The listing builds one solid part. Answer for the finished solid, in the listing's coordinates (mm). A direction names the side the tool comes from. Coordinates: 2 decimals unless noted, no trailing zeros. Order: outer loops, then holes, each group sorted by start corner. A loop starts at its lowest first (then second) coordinate and runs counter-clockwise, first axis right, second up. Notation, with made-up numbers: (-15.5, -28) -> (43.5, -28) arc R32 ccw to (43.5, 7) -> close; hole circle Ø5 at (11, 12). An arc over 180 degrees is marked (long way). Write each question's results on one line, items separated by ' | '. Start each with the question number.
(1) A tool of negligible diameter and unlimited length cuts with its end or side. For faces 4 (the face through (16, -21, 10)), 5 (the face through (9.15, -4.86, 15.1)), 6 (the face through (16.9, 4.14, 9.86)), from which of +Z, -Z, +X, -X, +Y, -Y can it reach the whole face along a straight path? Write none if from no direction.
(2) The part is cut by section C-C, the plane z = 10. Count the separate pieces of the cut face and the enclosed holes in it, then the cut area to 3 significant figures.
(3) Straight lines are drawn through the part: L1, parallel to X at y = 1, z = 2; L2, parallel to X at y = -7, z = 14; L3, parallel to Y at x = 3.75, z = -2.5. For each, find the intervals that lie inside material, in ascending order.
(4) The part is cut by section B-B, the plane x = 11.5. Give the vertices of the cut face in (y, z), then the cut area to 3 significant figures.
(5) Determine the mould class of faces 1 (the face through (2.768, -9.84, 13.646)), 2 (the face through (14.9, -4.86, 2.67)), 3 (the face through (13, -10, 20)) for opening direction Z: +Z half, -Z half, draft (parallel to the pull), parting line (faces both ways), or undercut.
(6) The part is cut by section A-A, the plane x = 20. Give the vertices of the cut face in (y, z), then the cut area to 3 significant figures.
(7) Given pin 1 (3 mm diameter, centred on x = 8, y = -19, fed in from -Z); pin 2 (5 mm diameter, centred on y = -14, z = 19, fed in from +X); pin 3 (1 mm diameter, centred on x = 20.5, z = 6.5, fed in from -Y), each flat-ended and moving along its own axis, determine where each tip first touches the part or whether it passes through.
```python
from build123d import *

# Parameters (mm, degrees)
SKETCH1_W           = 20
SKETCH1_H           = 20
BOSS_EXTRUDE1_DEPTH = 4
SKETCH2_R           = 3.65
CUT_EXTRUDE1_DEPTH  = 2.5
SKETCH3_R           = 2.25
CUT_EXTRUDE2_DEPTH  = 29.394541729
SKETCH4_W           = 12
SKETCH4_H           = 4
BOSS_EXTRUDE2_DEPTH = 10
SKETCH7_W           = 20
SKETCH7_H           = 4
BOSS_EXTRUDE3_DEPTH = 10
SKETCH8_W           = 8
SKETCH8_H           = 20
BOSS_EXTRUDE4_DEPTH = 5
SKETCH9_W           = 8
SKETCH9_H           = 20
BOSS_EXTRUDE5_DEPTH = 5
SKETCH10_R          = 1.6
CUT_EXTRUDE5_DEPTH  = 41.012498047
SKETCH11_W          = 32
SKETCH11_H          = 32
SKETCH11_W_2        = 20
SKETCH11_H_2        = 20
BOSS_EXTRUDE6_DEPTH = 6
FILLET6_R           = 3
SKETCH13_R          = 1.35
CUT_EXTRUDE7_DEPTH  = 6
FILLET7_R           = 3
FILLET13_R          = 2
FILLET14_SIZE       = 13


with BuildPart() as part:
    # Sketch1 → Boss-Extrude1 (new body)
    with BuildSketch(Plane(origin=(0, 0, 0), x_dir=(0, 0, -1), z_dir=(1, 0, 0))):
        with Locations((-10, -10)):
            Rectangle(SKETCH1_W, SKETCH1_H)
    extrude(amount=BOSS_EXTRUDE1_DEPTH)

    # Sketch2 → Cut-Extrude1 (cut)
    with BuildSketch(Plane(origin=(4, 0, 0), x_dir=(0, 0, -1), z_dir=(1, 0, 0))):
        with Locations((-10, -10)):
            Circle(SKETCH2_R)
    extrude(amount=-CUT_EXTRUDE1_DEPTH, mode=Mode.SUBTRACT)

    # Sketch3 → Cut-Extrude2 (cut, through all)
    with BuildSketch(Plane(origin=(1.5, 0, 0), x_dir=(0, 0, -1), z_dir=(1, 0, 0))):
        with Locations((-10, -10)):
            Circle(SKETCH3_R)
    extrude(amount=-CUT_EXTRUDE2_DEPTH, mode=Mode.SUBTRACT)

    # Sketch4 → Boss-Extrude2 (add)
    with BuildSketch(Plane(origin=(4, 0, 0), x_dir=(0, 0, -1), z_dir=(1, 0, 0))):
        Polygon((-20, 0), (-20, -20), (-16, -20), (-16, -16), (-16, -4), (-16, 0), align=None)
        with Locations((-10, -18)):
            Rectangle(SKETCH4_W, SKETCH4_H)
        Polygon((-4, -16), (-4, -20), (0, -20), (0, -4), (-4, -4), align=None)
        Polygon((0, 0), (-16, 0), (-16, -4), (-4, -4), (0, -4), align=None)
    extrude(amount=BOSS_EXTRUDE2_DEPTH)

    # Sketch7 → Boss-Extrude3 (add)
    with BuildSketch(Plane(origin=(14, 0, 0), x_dir=(0, 0, -1), z_dir=(1, 0, 0))):
        with Locations((-10, -18)):
            Rectangle(SKETCH7_W, SKETCH7_H)
        with Locations((-10, -2)):
            Rectangle(SKETCH7_W, SKETCH7_H)
    extrude(amount=BOSS_EXTRUDE3_DEPTH)

    # Sketch8 → Boss-Extrude4 (add)
    with BuildSketch(Plane(origin=(0, -20, 0), x_dir=(-1, 0, 0), z_dir=(0, -1, 0))):
        with Locations((-20, -10)):
            Rectangle(SKETCH8_W, SKETCH8_H)
    extrude(amount=BOSS_EXTRUDE4_DEPTH)

    # Sketch9 → Boss-Extrude5 (add)
    with BuildSketch(Plane(origin=(0, 0, 0), x_dir=(1, 0, 0), z_dir=(0, 1, 0))):
        with Locations((20, -10)):
            Rectangle(SKETCH9_W, SKETCH9_H)
    extrude(amount=BOSS_EXTRUDE5_DEPTH)

    # Sketch10 → Cut-Extrude5 (cut, through all)
    with BuildSketch(Plane(origin=(0, 0, 0), x_dir=(-1, 0, 0), z_dir=(0, 0, -1))):
        with Locations(Location((-20, 1, 0), (0, 0, 90))):
            Circle(SKETCH10_R)
        with Locations(Location((-20, -21, 0), (0, 0, 90))):
            Circle(SKETCH10_R)
    extrude(amount=-CUT_EXTRUDE5_DEPTH, mode=Mode.SUBTRACT)

    # Sketch11 → Boss-Extrude6 (add)
    with BuildSketch(Plane.ZY):
        with Locations((10, -10)):
            Rectangle(SKETCH11_W, SKETCH11_H)
        with Locations((10, -10)):
            Rectangle(SKETCH11_W_2, SKETCH11_H_2, mode=Mode.SUBTRACT)
    extrude(amount=-BOSS_EXTRUDE6_DEPTH)

    # Fillet6
    fillet6_edges = [part.edges().sort_by_distance(p)[0] for p in [
        (24, -16, 10),
        (24, -4, 10),
        (24, -25, 10),
        (16, -25, 10),
        (24, 5, 10),
        (16, 5, 10),
    ]]
    fillet(fillet6_edges, radius=FILLET6_R)

    # Sketch13 → Cut-Extrude7 (cut)
    with BuildSketch(Plane.ZY):
        with Locations((22.5, -10)):
            Circle(SKETCH13_R)
        with Locations((10, 2.5)):
            Circle(SKETCH13_R)
        with Locations((-2.5, -10)):
            Circle(SKETCH13_R)
        with Locations((10, -22.5)):
            Circle(SKETCH13_R)
    extrude(amount=-CUT_EXTRUDE7_DEPTH, mode=Mode.SUBTRACT)

    # Fillet7
    fillet7_edges = [part.edges().sort_by_distance(p)[0] for p in [
        (9, -4, 16),
        (9, -4, 4),
        (9, -16, 4),
        (9, -16, 16),
        (14, -16, 18),
        (14, -16, 2),
        (14, -4, 2),
        (14, -4, 18),
    ]]
    fillet(fillet7_edges, radius=FILLET7_R)

    # Fillet13
    fillet13_edges = [part.edges().sort_by_distance(p)[0] for p in [
        (11, 0, 20),
        (11, 0, 0),
    ]]
    fillet(fillet13_edges, radius=FILLET13_R)

    # Fillet14
    # a fillet whose section is not a circle: 13 mm, written as the material it takes off along each edge
    with BuildSketch(Plane(origin=(0, -26, -6), x_dir=(0, 1, 0), z_dir=(1, 0, 0)), Plane(origin=(0, -26, 26), x_dir=(0, 0, -1), z_dir=(1, 0, 0))) as fillet14_piece_1:
        with BuildLine():
            Bezier((FILLET14_SIZE, 0), (0, 0), (0, FILLET14_SIZE), weights=[1, 0.333333333, 1])
            Line((0, FILLET14_SIZE), (-FILLET14_SIZE * 0.02, FILLET14_SIZE))
            Line((-FILLET14_SIZE * 0.02, FILLET14_SIZE), (-FILLET14_SIZE * 0.02, -FILLET14_SIZE * 0.02))
            Line((-FILLET14_SIZE * 0.02, -FILLET14_SIZE * 0.02), (FILLET14_SIZE, -FILLET14_SIZE * 0.02))
            Line((FILLET14_SIZE, -FILLET14_SIZE * 0.02), (FILLET14_SIZE, 0))
        make_face()
    extrude(amount=6, mode=Mode.SUBTRACT)
    with BuildSketch(Plane(origin=(0, 6, -6), x_dir=(0, -1, 0), z_dir=(1, 0, 0)), Plane(origin=(0, 6, 26), x_dir=(0, 0, -1), z_dir=(1, 0, 0))) as fillet14_piece_2:
        with BuildLine():
            Bezier((FILLET14_SIZE, 0), (0, 0), (0, -FILLET14_SIZE), weights=[1, 0.333333333, 1])
            Line((0, -FILLET14_SIZE), (-FILLET14_SIZE * 0.02, -FILLET14_SIZE))
            Line((-FILLET14_SIZE * 0.02, -FILLET14_SIZE), (-FILLET14_SIZE * 0.02, FILLET14_SIZE * 0.02))
            Line((-FILLET14_SIZE * 0.02, FILLET14_SIZE * 0.02), (FILLET14_SIZE, FILLET14_SIZE * 0.02))
            Line((FILLET14_SIZE, FILLET14_SIZE * 0.02), (FILLET14_SIZE, 0))
        make_face()
    extrude(amount=6, mode=Mode.SUBTRACT)


solid = part.part
```
Established:
1) face 4: +Z, -Z, -Y | face 5: +X | face 6: +Z, -Z, +Y
2) separate pieces: 4 | enclosed holes: 2 | area: 307 mm^2
3) L1: x = 0 to 6, 16 to 18.4, 21.6 to 24 | L2: x = 0 to 4 | L3: y = -19.64 to -11.35, -8.65 to -0.36
4) outline: (-20, 0) -> (-2, 0) arc R2 ccw to (0, 2) -> (0, 18) arc R2 ccw to (-2, 20) -> (-20, 20) -> close; hole (-16, 7) arc R3 ccw to (-13, 4) -> (-7, 4) arc R3 ccw to (-4, 7) -> (-4, 13) arc R3 ccw to (-7, 16) -> (-13, 16) arc R3 ccw to (-16, 13) -> close | area: 262 mm^2
5) face 1: undercut | face 2: draft | face 3: +Z half
6) outline: (-25, 0) -> (-22.6, 0) -> (-22.6, 20) -> (-25, 20) -> close; (-19.4, 0) -> (-16, 0) -> (-16, 20) -> (-19.4, 20) -> close; (-4, 0) -> (-0.6, 0) -> (-0.6, 20) -> (-4, 20) -> close; (2.6, 0) -> (5, 0) -> (5, 20) -> (2.6, 20) -> close | area: 232 mm^2
7) pin 1: stops at z = 0 | pin 2: stops at x = 22.66 | pin 3: stops at y = -25
